CAD build for the part. Positions are in the model's coordinates, mm. A direction names the side the tool comes from. Give positions to 0.01 mm unless a question says otherwise; leave off trailing zeros. Order: outer loops, then holes, each group sorted by start corner. A loop starts at its lowest first (then second) coordinate and runs counter-clockwise, first axis right, second up. Notation, with made-up numbers: (29.25, 29) -> (56.25, 29) arc R26 cw to (56.25, 49) -> close; hole circle Ø6 at (13, -12). An arc over 180 degrees is marked (long way). Answer as CSV lines item,"result".
```python
from build123d import *

# Parameters (mm, degrees)
BOSS_EXTRUDE1_DEPTH             = 20
M3X0_5_TAPPED_HOLE1_D           = 2.5
M3X0_5_TAPPED_HOLE1_DEPTH       = 8.5
M3X0_5_TAPPED_HOLE1_CSINK_D     = 3.05
M3X0_5_TAPPED_HOLE1_CSINK_ANGLE = 90
M3X0_5_TAPPED_HOLE1_TIP         = 0.751075774
SKETCH4_R                       = 1.5
BOSS_EXTRUDE2_DEPTH             = 6


with BuildPart() as part:
    # Sketch1 → Boss-Extrude1 (new body)
    with BuildSketch(Plane(origin=(0, 0, 0), x_dir=(1, 0, 0), z_dir=(0, 1, 0))):
        Polygon((2.886751346, 0), (1.443375673, 2.5), (-1.443375673, 2.5), (-2.886751346, 0), (-1.443375673, -2.5), (1.443375673, -2.5), align=None)
    extrude(amount=BOSS_EXTRUDE1_DEPTH)

    # M3x0.5 Tapped Hole1
    with Locations(Plane(origin=(0, 20, 0), x_dir=(1, 0, 0), z_dir=(0, 1, 0))):
        with Locations((0, 0)):
            CounterSinkHole(M3X0_5_TAPPED_HOLE1_D / 2, M3X0_5_TAPPED_HOLE1_CSINK_D / 2, depth=M3X0_5_TAPPED_HOLE1_DEPTH, counter_sink_angle=M3X0_5_TAPPED_HOLE1_CSINK_ANGLE)
            with Locations((0, 0, -(M3X0_5_TAPPED_HOLE1_DEPTH + M3X0_5_TAPPED_HOLE1_TIP / 2))):  # 118° drill point
                Cone(0, M3X0_5_TAPPED_HOLE1_D / 2, M3X0_5_TAPPED_HOLE1_TIP, mode=Mode.SUBTRACT)

    # Sketch4 → Boss-Extrude2 (add)
    with BuildSketch(Plane.XZ):
        with Locations(Location((0, 0, 0), (0, 0, 90))):
            Circle(SKETCH4_R)
    extrude(amount=BOSS_EXTRUDE2_DEPTH)


solid = part.part
```
1) Which spindle directions (+Z, -Z, +X, -X, +Y, -Y) get a long thin tool onto all of the face, cutting with end or side? Do faces 4 (the flat face through (-2.155, 9.86, -1.267)), 5 (the cylindrical face through (-0.45, -2.96, 1.43)), 6 (the cylindrical face through (0.27, 15.55, 1.22)). Say none if no direction does.
Data:
face 4,"-Z, -X, +Y, -Y"
face 5,"-Y"
face 6,"+Y"
2) Band-saw the part on B-B, the plane x = 1.95. Write the cut outline in (y, z).
Data:
outline,"(0, -1.62) -> (20, -1.62) -> (20, 1.62) -> (0, 1.62) -> close"
3) Band-saw the part on A-A, the plane y = -3. Write the cut outline in (x, z).
Data:
outline,"circle Ø3 at (0, 0)"
4) Wall check: line 1 along Z through (x, y) = (0, 16.5); line 2 along Y through (x, z) = (2.45, -0.4); line 3 along X through (y, z) = (12.75, -0.25). Give the ranges that are in metal, low to high. Write a range as [from, to].
Data:
line 1,"z = [-2.5, -1.25], [1.25, 2.5]"
line 2,"y = [0, 20]"
line 3,"x = [-2.74, -1.22], [1.22, 2.74]"
5) Band-saw the part on C-C, the plane z = 1.85. Write the cut outline in (x, y).
Data:
outline,"(-1.82, 0) -> (1.82, 0) -> (1.82, 20) -> (-1.82, 20) -> close"
6) Pin check, flat tip, straight feed: P1, Ø3, axis at x = 0, z = 0, coming from the +Y side (3 decimals). Stop position of the tip, or through.
Data:
P1,"stops at y = 19.975"
7) Pull direction Z, two halves, no side cores. Call faces 1 (the flat face through (-2.175, 9.86, 1.233)), 2 (the flat face through (0, 10, -2.5)), 3 (the conical face through (-0.05, 10.88, 0.21)): pulls with the +Z half, pulls with the -Z half, needs draft (parallel to the pull), parting line crosses it, or undercut.
Data:
face 1,"pulls with the +Z half"
face 2,"pulls with the -Z half"
face 3,"undercut"
